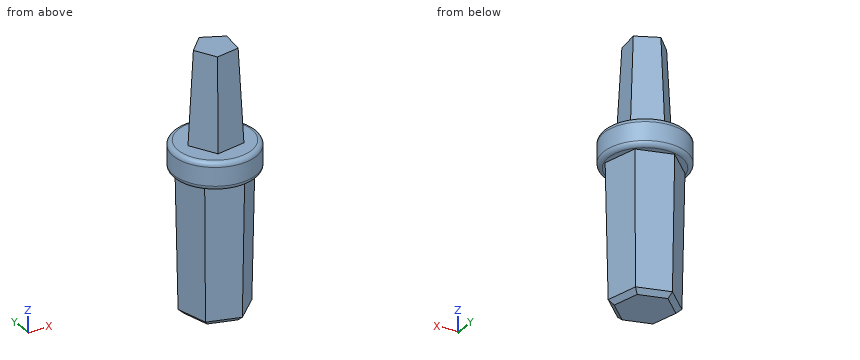
from build123d import *

# Parameters (mm, degrees)
F1_DEPTH = 10
F1_TAPER = 2.56
F2_R     = 4.5
F3_DEPTH = 3
F4_R     = 0.5
F6_DEPTH = 15
F6_TAPER = 1
F7_SIZE  = 0.5


with BuildPart() as f1:
    # F0 (on Top) → F1 (new body)
    with BuildSketch(Plane.XY):
        Polygon((-1.173613, -2.502389), (2.017247, -1.889453), (2.42034, 1.334643), (-0.521395, 2.714308), (-2.74258, 0.342891), align=None)
    extrude(amount=F1_DEPTH, taper=F1_TAPER)

    # F2 (on Top) → F3 (join)
    with BuildSketch(Plane.XY):
        Circle(F2_R)
    extrude(amount=-F3_DEPTH)

    # F4
    f4_edges = [f1.edges().sort_by_distance(p)[0] for p in [
        (-4.5, 0, 0),
        (-4.5, 0, -3),
    ]]
    fillet(f4_edges, radius=F4_R)

    # F5 (on face) → F6 (join)
    with BuildSketch(Plane(origin=(0, 0, -3), x_dir=(1, 0, 0), z_dir=(0, 0, -1))):
        Polygon((2.770276, -2.707296), (3.729724, 1.045481), (0.959449, 3.752777), (-2.770276, 2.707296), (-3.729724, -1.045481), (-0.959449, -3.752777), align=None)
    extrude(amount=F6_DEPTH, taper=F6_TAPER)

    # F7
    f7_edges = [f1.edges().sort_by_distance(p)[0] for p in [
        (2.161589, -2.211874, -18),
        (-0.834745, -2.977927, -18),
        (-2.996333, -0.766054, -18),
        (-2.161589, 2.211874, -18),
        (0.834745, 2.977927, -18),
        (2.996333, 0.766054, -18),
    ]]
    chamfer(f7_edges, length=F7_SIZE)


solid = f1.part
Model file for the job. Use its own axes, mm. Give positions to 0.01 mm unless a question says otherwise; leave off trailing zeros. Loops run counter-clockwise (first coordinate to the right, second up) from the corner with the lowest first, then second, coordinate; pieces in that order, holes last.
1) Flat gauge pins, fed straight in: pin 1 Ø3 at (y, z) = (-3.5, 6.5) entering from -X; pin 2 Ø1.5 at (x, z) = (-0.5, -7) entering from +Y; pin 3 Ø2 at (x, z) = (1, 5) entering from +Y. Where does each tip first touch, or does it go through?
2) Saw through at B-B (z = -2). Write the cut outline in (x, y).
3) Saw through at A-A (z = 7). Write the cut outline in (x, y) (3 decimals), plus the area to 3 significant figures.
4) Saw through at C-C (z = 2.5). Write the cut outline in (x, y) (3 decimals), plus the area to 3 significant figures.
5) Wall check: line 1 (Z direction, x = -2, y = 1.5); line 2 (X direction, y = 2.5, z = -8.75); line 3 (Z direction, x = -3.75, y = -1.5). Give the ranges that are in metal, low to high.
Answer block:
1. pin 1: stops at x = -1.12
1. pin 2: stops at y = 3.69
1. pin 3: stops at y = 2.23
2. outline: circle Ø9 at (0, 0)
3. outline: (-2.359, 0.295) - (-1.009, -2.152) - (1.735, -1.625) - (2.082, 1.148) - (-0.448, 2.334) - close
3. area: 13.4 mm2
4. outline: (-2.605, 0.326) - (-1.115, -2.377) - (1.916, -1.795) - (2.299, 1.268) - (-0.495, 2.579) - close
4. area: 16.4 mm2
5. line 1: z = -18 to 0
5. line 2: x = -2.1 to 2.72
5. line 3: z = -3 to 0
